The model under review builds one solid part; all positions refer to its coordinate system, in mm. A direction names the side the tool comes from. Round coordinates to 2 decimals unless told otherwise and drop trailing zeros. Write each loop counter-clockwise with the first axis right and the second up, starting at its lowest first coordinate (ties: lowest second). Pieces come first, ordered by that corner, then holes. Notation, with made-up numbers: (7.5, -26) - (41.5, -26) arc R26 ccw to (41.5, 10) - close; hole circle Ø6 at (87.25, -14). An arc over 180 degrees is marked (long way). One line per question, with ' | ' between items. Start each with the question number.
```python
from build123d import *

# Parameters (mm, degrees)
BOSS_EXTRUDE1_DEPTH = 4
SKETCH2_R           = 5
BOSS_EXTRUDE2_DEPTH = 20
SKETCH3_R           = 2
CUT_EXTRUDE1_DEPTH  = 10
SKETCH4_R           = 1.5
CUT_EXTRUDE2_DEPTH  = 7
SKETCH5_R           = 1.5
CUT_EXTRUDE3_DEPTH  = 10


with BuildPart() as part:
    # Sketch1 → Boss-Extrude1 (new body)
    with BuildSketch(Plane.XY):
        Polygon((0, 6.92820323), (-6, 3.464101615), (-6, -3.464101615), (0, -6.92820323), (6, -3.464101615), (6, 3.464101615), align=None)
    extrude(amount=BOSS_EXTRUDE1_DEPTH)

    # Sketch2 → Boss-Extrude2 (add)
    with BuildSketch(Plane.XY.offset(4)):
        Circle(SKETCH2_R)
    extrude(amount=BOSS_EXTRUDE2_DEPTH)

    # Sketch3 → Cut-Extrude1 (cut)
    with BuildSketch(Plane.XY.offset(24)):
        Circle(SKETCH3_R)
    extrude(amount=-CUT_EXTRUDE1_DEPTH, mode=Mode.SUBTRACT)

    # Sketch4 → Cut-Extrude2 (cut)
    with BuildSketch(Plane(origin=(0, 0, 0), x_dir=(0, 0, -1), z_dir=(1, 0, 0))):
        with Locations((-18.5, 0)):
            Circle(SKETCH4_R)
    extrude(amount=CUT_EXTRUDE2_DEPTH, mode=Mode.SUBTRACT)

    # Sketch5 → Cut-Extrude3 (cut)
    with BuildSketch(Plane(origin=(0, 0, 0), x_dir=(-1, 0, 0), z_dir=(0, 0, -1))):
        Circle(SKETCH5_R)
    extrude(amount=-CUT_EXTRUDE3_DEPTH, mode=Mode.SUBTRACT)


solid = part.part
```
1. The part is to be moulded in two halves that separate along Z. For faces 4 (the face through (0, 0, 14)), 5 (the face through (3.1, -0.9, 19.7)), 6 (the face through (-2, 0, 19)), say which applies: pulls with the +Z half, pulls with the -Z half, needs draft (parallel to the pull), parting line crosses it, or undercut.
2. Add section D-D, the plane x = 0.5. Write out the cut boundary in (y, z), then the cut area to 3 significant figures.
3. Add section C-C, the plane z = 7. Write out the cut boundary in (x, y).
4. Clearance check with flat-ended pins moving along their axes: P1, Ø5, axis at y = 3.5, z = 20.5, coming from the -X side; P2, Ø2, axis at x = 0, y = 0, coming from the +Z side; P3, Ø0.9, axis at x = 0.5, y = 0.5, coming from the -Z side. State where each tip first meets the part, or that it passes through.
5. Add section A-A, the plane y = 0. Write out the cut boundary in (x, z), then the cut area to 3 significant figures.
6. Wall thickness on line 1 along Y through (x, z) = (0, 19.25); line 2 along Y through (x, z) = (0, 4.5); line 3 along X through (y, z) = (1.75, 20.25): over which ranges is each line inside the solid? List them lowest first. Write a range as [from, to].
7. Machinability: for faces 1 (the face through (0, 0, 10)), 2 (the face through (6, 0, 2)), 3 (the face through (-0.9, -5.1, 4)), which of the approach directions +Z, -Z, +X, -X, +Y, -Y give a long, thin tool a straight path to every point of the face, cutting with its end or side? Answer none if there is none.
8. Add section B-B, the plane x = 3.25. Write out the cut boundary in (y, z).
Geometry check:
1) face 4: pulls with the +Z half | face 5: undercut | face 6: needs draft
2) outline: (-6.64, 0) - (-1.41, 0) - (-1.41, 10) - (1.41, 10) - (1.41, 0) - (6.64, 0) - (6.64, 4) - (4.97, 4) - (4.97, 24) - (1.94, 24) - (1.94, 14) - (-1.94, 14) - (-1.94, 24) - (-4.97, 24) - (-4.97, 4) - (-6.64, 4) - close | area: 185 mm2
3) outline: circle Ø10 at (0, 0); hole circle Ø3 at (0, 0)
4) P1: stops at x = -4.9 | P2: stops at z = 14 | P3: stops at z = 10
5) outline: (-6, 0) - (-1.5, 0) - (-1.5, 10) - (1.5, 10) - (1.5, 0) - (6, 0) - (6, 4) - (5, 4) - (5, 17) - (2, 17) - (2, 14) - (-2, 14) - (-2, 24) - (-5, 24) - (-5, 4) - (-6, 4) - close; (2, 20) - (5, 20) - (5, 24) - (2, 24) - close | area: 169 mm2
6) line 1: y = [-5, -2], [2, 5] | line 2: y = [-5, -1.5], [1.5, 5] | line 3: x = [-4.68, -0.97], [0.97, 4.68]
7) face 1: -Z | face 2: +Z, -Z, +X, +Y, -Y | face 3: +Z
8) outline: (-5.05, 0) - (5.05, 0) - (5.05, 4) - (3.8, 4) - (3.8, 24) - (-3.8, 24) - (-3.8, 4) - (-5.05, 4) - close; hole circle Ø3 at (0, 18.5)
